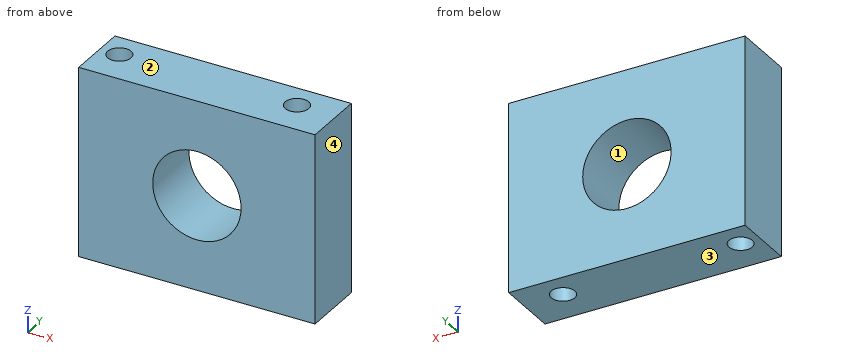
from build123d import *

# Parameters (mm, degrees)
F0_W     = 95.25
F0_H     = 76.2
F0_R     = 17.812688
F1_DEPTH = 25.4
F2_R     = 4.71978
F2_R_2   = 4.777232
F3_DEPTH = 254
F4_DEPTH = 254


with BuildPart() as f1:
    # F0 (on Front) → F1 (new body)
    with BuildSketch(Plane.XZ):
        with Locations((10.070114, 0)):
            Rectangle(F0_W, F0_H)
        with Locations((10.070114, 0)):
            Circle(F0_R, mode=Mode.SUBTRACT)
    extrude(amount=F1_DEPTH)

    # F2 (on face) → F3 (cut)
    with BuildSketch(Plane.XY.offset(38.1)):
        with Locations((-29.710518, -10.510667)):
            Circle(F2_R)
        with Locations((41.842777, -10.510667)):
            Circle(F2_R_2)
    extrude(amount=-F3_DEPTH, mode=Mode.SUBTRACT)

    # F2 (on face) → F4 (cut)
    with BuildSketch(Plane.XY.offset(38.1)):
        with Locations((-29.710518, -10.510667)):
            Circle(F2_R)
        with Locations((41.842777, -10.510667)):
            Circle(F2_R_2)
    extrude(amount=-F4_DEPTH, mode=Mode.SUBTRACT)


solid = f1.part
Here's how the part is built. I have some questions about the finished solid (model axes, mm). Face numbers are marked on the shaded views. Coordinates: 2 decimals unless noted, no trailing zeros. Order: outer loops, then holes, each group sorted by start corner. A loop starts at its lowest first (then second) coordinate and runs counter-clockwise, first axis right, second up.
Item 1: If we section it at A-A on z = -13.5: List the corners of the cut face in (x, y) for me.
Result sheet:
outline: (-37.55, -25.4) - (-1.55, -25.4) - (-1.55, 0) - (-37.55, 0) - close; (21.69, -25.4) - (57.7, -25.4) - (57.7, 0) - (21.69, 0) - close; hole circle Ø9.44 at (-29.71, -10.51); hole circle Ø9.55 at (41.84, -10.51)
Item 2: If we section it at C-C on y = -20.25: List the corners of the cut face in (x, z) for me.
Result sheet:
outline: (-37.55, -38.1) - (57.7, -38.1) - (57.7, 38.1) - (-37.55, 38.1) - close; hole circle Ø35.63 at (10.07, 0)
Item 3: If we section it at D-D on x = -6: List the corners of the cut face in (y, z) for me.
Result sheet:
outline: (-25.4, -38.1) - (0, -38.1) - (0, -7.68) - (-25.4, -7.68) - close; (-25.4, 7.68) - (0, 7.68) - (0, 38.1) - (-25.4, 38.1) - close
Item 4: I need wall thicknesses on line 1 (Y direction, x = -30, z = -33.5); line 2 (X direction, y = -7.5, z = -25.5); line 3 (X direction, y = -8.25, z = -11.5). Which ranges of each line are inside material? Lowest first, please.
Result sheet:
line 1: y = -25.4 to -15.22, -5.8 to 0
line 2: x = -37.55 to -33.35, -26.08 to 38.13, 45.55 to 57.7
line 3: x = -37.55 to -33.85, -25.57 to -3.53, 23.67 to 37.63, 46.05 to 57.7
Item 5: If we mould it in two halves opening along Z, with no side actions, what happens to the marked faces 1, 2, 3 and 4? For each: +Z half, -Z half, draft (parallel to the pull), parting line (faces both ways), or undercut.
Result sheet:
face 1: undercut
face 2: +Z half
face 3: -Z half
face 4: draft
Item 6: If we section it at B-B on y = -9: List the corners of the cut face in (x, z) for me.
Result sheet:
outline: (-37.55, -38.1) - (-34.18, -38.1) - (-34.18, 38.1) - (-37.55, 38.1) - close; (-25.24, -38.1) - (37.31, -38.1) - (37.31, 38.1) - (-25.24, 38.1) - close; (46.37, -38.1) - (57.7, -38.1) - (57.7, 38.1) - (46.37, 38.1) - close; hole circle Ø35.63 at (10.07, 0)
